Geometry: final body of the model. Coordinates: model frame, mm. Coordinates: 2 decimals unless noted, no trailing zeros. Order: outer loops, then holes, each group sorted by start corner. A loop starts at its lowest first (then second) coordinate and runs counter-clockwise, first axis right, second up. Notation, with made-up numbers: M 33.25,-38.75 L 48.25,-38.75 A31 cw 48.25,0.25 Z; hole C 49,-4 d6. An arc over 180 degrees is marked long. Write item = value, one per line.
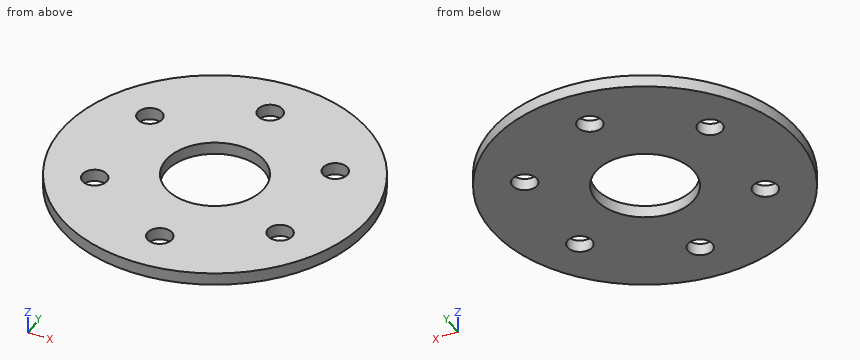
from build123d import *

# Parameters (mm, degrees)
SKETCH1_R               = 12.5
BOSS_EXTRUDE1_DEPTH     = 1
CUT_EXTRUDE2_START      = -2
SKETCH2_R               = 1
CUT_EXTRUDE2_DEPTH      = 20.70593121
CIRPATTERN1_COUNT       = 6
CUT_EXTRUDE3_DEPTH      = 18.70593121
CUT_EXTRUDE3_DEPTH_BACK = 18.70593121
SKETCH4_R               = 4


with BuildPart() as part:
    # Sketch1 → Boss-Extrude1 (new body)
    with BuildSketch(Plane.XY):
        Circle(SKETCH1_R)
    extrude(amount=BOSS_EXTRUDE1_DEPTH)

    # Sketch2 → Cut-Extrude2 (cut)
    with BuildSketch(Plane.XY.offset(CUT_EXTRUDE2_START)):
        with Locations((0, 8.75)):
            Circle(SKETCH2_R)
    cut_extrude2 = extrude(amount=CUT_EXTRUDE2_DEPTH, mode=Mode.SUBTRACT)

    # CirPattern1: Cut-Extrude2 ×6 about axis
    cirpattern1_axis = Axis((0, 0, 0), (0, 0, 1))
    for i in range(1, CIRPATTERN1_COUNT):
        add(cut_extrude2.rotate(cirpattern1_axis, i * 360 / CIRPATTERN1_COUNT), mode=Mode.SUBTRACT)

    # Sketch4 → Cut-Extrude3 (cut, two sides: drawn at the far end of the back side and taken through both)
    with BuildSketch(Plane(origin=(0, 0, 0), x_dir=(-1, 0, 0), z_dir=(0, 0, -1)).offset(-CUT_EXTRUDE3_DEPTH_BACK)):
        Circle(SKETCH4_R)
    extrude(amount=CUT_EXTRUDE3_DEPTH + CUT_EXTRUDE3_DEPTH_BACK, mode=Mode.SUBTRACT)


solid = part.part
1) Section C-C, the plane x = 3. Return loops of the section in (y, z), and give its area (3 significant figures).
Numbers:
outline = M -12.13,0 L -2.65,0 L -2.65,1 L -12.13,1 Z; M 2.65,0 L 12.13,0 L 12.13,1 L 2.65,1 Z
area = 19.0 mm²
2) Section D-D, the plane z = 0.5. Return loops of the section in (x, y) (3 decimals), and give its area (3 significant figures).
Numbers:
outline = C 0,0 d25; hole C -7.578,-4.375 d2; hole C -7.578,4.375 d2; hole C 0,0 d8; hole C 0,-8.75 d2; hole C 0,8.75 d2; hole C 7.578,-4.375 d2; hole C 7.578,4.375 d2
area = 422 mm²
3) Line query: L1, parallel to Y at x = 8, z = 0.2; L2, parallel to X at y = 4.5, z = 0.6; L3, parallel to Y at x = 0, z = 0.55. Output: solid intervals per line, ascending.
Numbers:
L1 = -9.6 to -5.28, -3.47 to 3.47, 5.28 to 9.6
L2 = -11.66 to -8.57, -6.59 to 6.59, 8.57 to 11.66
L3 = -12.5 to -9.75, -7.75 to -4, 4 to 7.75, 9.75 to 12.5
4) Section A-A, the plane y = 0. Return loops of the section in (x, z), and give its area (3 significant figures).
Numbers:
outline = M -12.5,0 L -4,0 L -4,1 L -12.5,1 Z; M 4,0 L 12.5,0 L 12.5,1 L 4,1 Z
area = 17.0 mm²
5) Pin query (flat end, axial travel): pin 1 (3 mm diameter, centred on x = -4.5, y = -1, fed in from -Z). Return the tip coordinate at first contact, or that it passes through.
Numbers:
pin_1 = 0
6) Section B-B, the plane x = 0. Return loops of the section in (y, z), and give its area (3 significant figures).
Numbers:
outline = M -12.5,0 L -9.75,0 L -9.75,1 L -12.5,1 Z; M -7.75,0 L -4,0 L -4,1 L -7.75,1 Z; M 4,0 L 7.75,0 L 7.75,1 L 4,1 Z; M 9.75,0 L 12.5,0 L 12.5,1 L 9.75,1 Z
area = 13.0 mm²
